from build123d import *

# Parameters (mm, degrees)
SKETCH1_R               = 1.75
BOSS_EXTRUDE1_DEPTH     = 7
SKETCH1_4_R             = 4
BOSS_EXTRUDE2_DEPTH     = 7
CUT_EXTRUDE1_DEPTH      = 92.744209627
CUT_EXTRUDE1_DEPTH_BACK = 92.744209627
SKETCH2_W               = 104
SKETCH2_H               = 76.59410066


with BuildPart() as part:
    # Sketch1 → Boss-Extrude1 (new body)
    with BuildSketch(Plane(origin=(0, 0, 0), x_dir=(0, 0, -1), z_dir=(1, 0, 0))):
        Polygon((-5, 11), (-10, 6), (-10, -6), (-5, -11), (30, -11), (30, -9), (90, -9), (90, 11), align=None)
        with Locations((34, 7)):
            Circle(SKETCH1_R, mode=Mode.SUBTRACT)
        with Locations((34, -5)):
            Circle(SKETCH1_R, mode=Mode.SUBTRACT)
        with BuildLine():
            Line((45, 6.75), (47, 6.75))
            ThreePointArc((47, 6.75), (48.75, 5), (47, 3.25))
            Line((47, 3.25), (45, 3.25))
            ThreePointArc((45, 3.25), (43.25, 5), (45, 6.75))
        make_face(mode=Mode.SUBTRACT)
        with BuildLine():
            Line((64, -3.25), (66, -3.25))
            ThreePointArc((66, -3.25), (67.75, -5), (66, -6.75))
            Line((66, -6.75), (64, -6.75))
            ThreePointArc((64, -6.75), (62.25, -5), (64, -3.25))
        make_face(mode=Mode.SUBTRACT)
        with BuildLine():
            Line((85, 3.25), (83, 3.25))
            ThreePointArc((83, 3.25), (81.25, 5), (83, 6.75))
            Line((83, 6.75), (85, 6.75))
            ThreePointArc((85, 6.75), (86.75, 5), (85, 3.25))
        make_face(mode=Mode.SUBTRACT)
    extrude(amount=BOSS_EXTRUDE1_DEPTH)

    # Sketch1_4 → Boss-Extrude2 (add)
    with BuildSketch(Plane(origin=(0, 0, 0), x_dir=(0, 0, -1), z_dir=(1, 0, 0))):
        Circle(SKETCH1_4_R)
    extrude(amount=-BOSS_EXTRUDE2_DEPTH)

    # Sketch2 → Cut-Extrude1 (cut, two sides: drawn at the far end of the back side and taken through both)
    with BuildSketch(Plane(origin=(7, 0, 0), x_dir=(0, 0, -1), z_dir=(1, 0, 0)).offset(-CUT_EXTRUDE1_DEPTH_BACK)):
        with Locations((90, -9)):
            Rectangle(SKETCH2_W, SKETCH2_H)
    extrude(amount=CUT_EXTRUDE1_DEPTH + CUT_EXTRUDE1_DEPTH_BACK, mode=Mode.SUBTRACT)


solid = part.part
The listing builds one solid part. Answer for the finished solid, in the listing's coordinates (mm). A direction names the side the tool comes from. Coordinates: 2 decimals unless noted, no trailing zeros. Order: outer loops, then holes, each group sorted by start corner. A loop starts at its lowest first (then second) coordinate and runs counter-clockwise, first axis right, second up. Notation, with made-up numbers: M 10,59 L 55,59 A28 cw 55,82 Z; hole C 6.25,61 d3. An arc over 180 degrees is marked long. Use CSV: the item, a comma, the result in double quotes.
Q1. Straight lines are drawn through the part: L1, parallel to Y at x = 4.75, z = -34; L2, parallel to X at y = 5.75, z = -4; L3, parallel to Z at x = 0.5, y = -10. For each, find the intervals that lie inside material, in ascending order.
Here are the results:
L1,"-9 to -6.75, -3.25 to 5.25, 8.75 to 11"
L2,"0 to 7"
L3,"-30 to 6"
Q2. Section D-D (z = -34) is taken. Determine the outline of the cut face in (x, y).
Here are the results:
outline,"M 0,-9 L 7,-9 L 7,-6.75 L 0,-6.75 Z; M 0,-3.25 L 7,-3.25 L 7,5.25 L 0,5.25 Z; M 0,8.75 L 7,8.75 L 7,11 L 0,11 Z"
Q3. Determine the mould class of faces 1 (the flat face through (3, -8, 8)), 2 (the flat face through (-7, 0, 0)), 3 (the flat face through (3, 1, -38)), 4 (the cylindrical face through (3.45, 5.94, -32.61)) for opening direction Z: pulls with the +Z half, pulls with the -Z half, needs draft (parallel to the pull), parting line crosses it, or undercut.
Here are the results:
face 1,"pulls with the +Z half"
face 2,"needs draft"
face 3,"pulls with the -Z half"
face 4,"undercut"
Q4. A tool of negligible diameter and unlimited length cuts with its end or side. For faces 5 (the flat face through (3, -10, -30)), 6 (the cylindrical face through (-3.451, -3.905, 0.867)), 7 (the cylindrical face through (3.45, -4.92, -32.25)), from which of +Z, -Z, +X, -X, +Y, -Y can it reach the whole face along a straight path? Write none if from no direction.
Here are the results:
face 5,"-Z, +X, -X, -Y"
face 6,"-X"
face 7,"+X, -X"
Q5. Section C-C (x = 5.75) is taken. Determine the outline of the cut face in (y, z), then the cut area to 3 significant figures.
Here are the results:
outline,"M -11,-30 L -9,-30 L -9,-38 L 11,-38 L 11,5 L 6,10 L -6,10 L -11,5 Z; hole C -5,-34 d3.5; hole C 7,-34 d3.5"
area,"996 mm2"
Q6. Given pin 1 Ø11 at (y, z) = (0.5, -14.5) entering from -X; pin 2 Ø2 at (x, y) = (2.5, -9.5) entering from -Z; pin 3 Ø2 at (x, z) = (2.5, -35.5) entering from -Y; pin 4 Ø2 at (y, z) = (-5, -34) entering from -X, each flat-ended and moving along its own axis, determine where each tip first touches the part or whether it passes through.
Here are the results:
pin 1,"x = 0"
pin 2,"z = -38"
pin 3,"y = -9"
pin 4,"through"
Q7. Section B-B (z = 0) is taken. Determine the outline of the cut face in (x, y).
Here are the results:
outline,"M -7,-4 L 0,-4 L 0,-11 L 7,-11 L 7,11 L 0,11 L 0,4 L -7,4 Z"
Q8. Section A-A (y = -5) is taken. Determine the outline of the cut face in (x, z), then the cut area to 4 significant figures.
Here are the results:
outline,"M 0,-38 L 7,-38 L 7,-35.75 L 0,-35.75 Z; M 0,-32.25 L 7,-32.25 L 7,10 L 0,10 Z"
area,"311.5 mm2"
